from build123d import *

# Parameters (mm, degrees)
SKETCH1_R      = 7
EXTRUDE1_DEPTH = 37
EXTRUDE5_START = -20
SKETCH5_R      = 9
EXTRUDE5_DEPTH = 4
EXTRUDE3_START = -4
EXTRUDE3_DEPTH = 36.127995093
SKETCH4_R      = 7
SKETCH4_R_2    = 6
EXTRUDE4_DEPTH = 10
SKETCH6_R      = 6
EXTRUDE6_DEPTH = 15
CHAMFER1_SIZE  = 0.3
SKETCH7_R      = 1.6
EXTRUDE7_DEPTH = 12
EXTRUDE8_START = -3.5
EXTRUDE8_DEPTH = 12
EXTRUDE9_START = 3.5
EXTRUDE9_DEPTH = 51.035035296


with BuildPart() as part:
    # Sketch1 → Extrude1 (new, symmetric)
    with BuildSketch(Plane.XY):
        Circle(SKETCH1_R)
    extrude(amount=EXTRUDE1_DEPTH, both=True)

    # Sketch5 → Extrude5 (add)
    with BuildSketch(Plane.XY.offset(37).offset(EXTRUDE5_START)):
        Circle(SKETCH5_R)
    extrude(amount=-EXTRUDE5_DEPTH)

    # Sketch3 → Extrude3 (cut, through all)
    with BuildSketch(Plane(origin=(0, 0, 0), x_dir=(1, 0, 0), z_dir=(0, 1, 0)).offset(EXTRUDE3_START)):
        with BuildLine():
            Line((-2.5, -27), (-2.5, -17))
            ThreePointArc((-2.5, -17), (0, -14.5), (2.5, -17))
            Line((2.5, -17), (2.5, -27))
            ThreePointArc((2.5, -27), (0, -29.5), (-2.5, -27))
        make_face()
    extrude(amount=-EXTRUDE3_DEPTH, mode=Mode.SUBTRACT)

    # Sketch4 → Extrude4 (cut)
    with BuildSketch(Plane.XY.offset(37)):
        Circle(SKETCH4_R)
        Circle(SKETCH4_R_2, mode=Mode.SUBTRACT)
    extrude4 = extrude(amount=-EXTRUDE4_DEPTH, mode=Mode.SUBTRACT)

    # Mirror1: Extrude4 across plane
    add(extrude4.mirror(Plane.XY), mode=Mode.SUBTRACT)

    # Sketch6 → Extrude6 (add)
    with BuildSketch(Plane.XY.offset(37)):
        Circle(SKETCH6_R)
    extrude6 = extrude(amount=EXTRUDE6_DEPTH)

    # Mirror2: Extrude6 across plane
    add(extrude6.mirror(Plane.XY))

    # Chamfer1
    chamfer1_edges = [part.edges().sort_by_distance(p)[0] for p in [
        (-6, 0, 52),
        (-6, 0, -52),
        (-7, 0, -27),
        (-9, 0, 13),
        (-5.408326913, 7.193747285, 17),
        (0, 7, 27),
    ]]
    chamfer(chamfer1_edges, length=CHAMFER1_SIZE)

    # Sketch7 → Extrude7 (cut)
    with BuildSketch(Plane.XY.offset(52)):
        Circle(SKETCH7_R)
    extrude7 = extrude(amount=-EXTRUDE7_DEPTH, mode=Mode.SUBTRACT)

    # Mirror3: Extrude7 across plane
    add(extrude7.mirror(Plane.XY), mode=Mode.SUBTRACT)

    # Sketch8 → Extrude8 (cut)
    with BuildSketch(Plane(origin=(0, 0, 0), x_dir=(1, 0, 0), z_dir=(0, 1, 0)).offset(EXTRUDE8_START)):
        with BuildLine():
            Line((2, 52), (2, 42))
            ThreePointArc((2, 42), (0, 40), (-2, 42))
            Line((-2, 42), (-2, 52))
            ThreePointArc((-2, 52), (0, 54), (2, 52))
        make_face()
    extrude(amount=-EXTRUDE8_DEPTH, mode=Mode.SUBTRACT)

    # Sketch9 → Extrude9 (cut, through all)
    with BuildSketch(Plane(origin=(0, 0, 0), x_dir=(1, 0, 0), z_dir=(0, 1, 0)).offset(EXTRUDE9_START)):
        with BuildLine():
            Line((-2, -52), (-2, -42))
            ThreePointArc((-2, -42), (0, -40), (2, -42))
            Line((2, -42), (2, -52))
            ThreePointArc((2, -52), (0, -54), (-2, -52))
        make_face()
    extrude(amount=EXTRUDE9_DEPTH, mode=Mode.SUBTRACT)


solid = part.part
CAD build for the part. Positions are in the model's coordinates, mm. A direction names the side the tool comes from. Coordinates: 2 decimals unless noted, no trailing zeros. Loops run counter-clockwise (first coordinate to the right, second up) from the corner with the lowest first, then second, coordinate; pieces in that order, holes last. Notation, with made-up numbers: (54, 31) - (68, 31) arc R16 cw to (68, 36) - close; hole circle Ø3 at (11.25, -6). An arc over 180 degrees is marked (long way). Use one line per item in the form item = value. Start each with the question number.
1) Tool access for faces 4 (the face through (-0.1, -6.5, 14.5)), 5 (the face through (-2, -5, -47)), 6 (the face through (0, 7.2, 17)), 7 (the face through (-6, 4, 13)): list every direction of +Z, -Z, +X, -X, +Y, -Y with a clear straight run to the whole face (end or side of a thin tool).
2) Flat gauge pins, fed straight in: pin 1 (6 mm diameter, centred on x = -4.5, y = 5.5, fed in from +Z); pin 2 (1.1 mm diameter, centred on y = 4.5, z = 49, fed in from +X); pin 3 (6 mm diameter, centred on x = 7, z = 22, fed in from +Y); pin 4 (1.2 mm diameter, centred on x = 0, z = 45, fed in from +Y). Where does each tip first touch, or does it go through?
3) Band-saw the part on A-A (z = -17). Give the cut face in (x, y).
4) Two-plate mould, pull along Z, no slides. Class faces 1 (the face through (0, -5, -40)), 2 (the face through (2.5, -5, 22)), 3 (the face through (2, 5, 47)): +Z half, -Z half, draft (parallel to the pull), parting line (faces both ways), or undercut.
5) Band-saw the part on B-B (z = -36.5). Give the cut face in (x, y), and give its area (3 significant figures).
6) Drill centre lines: L1, parallel to Y at x = 0, z = 44; L2, parallel to Y at x = 0, z = -47.5; L3, parallel to Z at x = -7.75, y = 3.75. Where is each one in solid material? Low to high. Write a range as from..to.
Check values:
q1.face_4 = -Y
q1.face_5 = -Z, -Y
q1.face_6 = +Z
q1.face_7 = -Z
q2.pin_1 = 52
q2.pin_2 = 4.52
q2.pin_3 = 5.74
q2.pin_4 = 3.5
q3.outline = circle Ø14 at (0, 0)
q4.face_1 = -Z half
q4.face_2 = undercut
q4.face_3 = draft
q5.outline = circle Ø12 at (0, 0)
q5.area = 113 mm2
q6.L1 = -6..-1.6, 1.6..3.5
q6.L2 = -3.5..-1.6, 1.6..6
q6.L3 = 13..17
